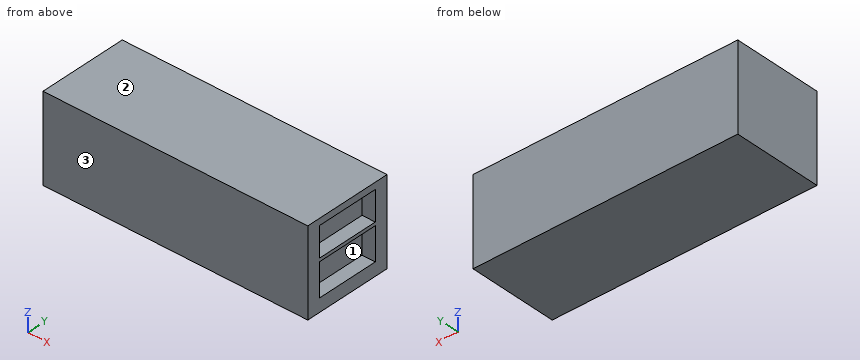
from build123d import *

# Parameters (mm, degrees)
F0_W     = 2032
F0_H     = 660.4
F1_DEPTH = 685.8
F2_W     = 482.6
F2_H     = 228.6
F2_H_2   = 254
F3_DEPTH = 101.6
F4_W     = 482.6
F4_H     = 254
F5_DEPTH = 101.6


with BuildPart() as f1:
    # F0 (on Front) → F1 (new body)
    with BuildSketch(Plane.XZ):
        with Locations((13.692988, -207.793446)):
            Rectangle(F0_W, F0_H)
    extrude(amount=F1_DEPTH)

    # F2 (on face) → F3 (cut)
    with BuildSketch(Plane.YZ.offset(1029.692988)):
        with Locations((-342.9, -42.693446)):
            Rectangle(F2_W, F2_H)
        with Locations((-342.9, -309.393446)):
            Rectangle(F2_W, F2_H_2)
    extrude(amount=-F3_DEPTH, mode=Mode.SUBTRACT)

    # F4 (on face) → F5 (join)
    with BuildSketch(Plane(origin=(-1002.307012, 0, 0), x_dir=(0, -1, 0), z_dir=(-1, 0, 0))):
        with Locations((342.9, -55.393446)):
            Rectangle(F4_W, F4_H)
        with Locations((342.9, -334.793446)):
            Rectangle(F4_W, F4_H)
    extrude(amount=-F5_DEPTH)


solid = f1.part
Geometry check sheet. Reference: the model listing, model coordinates, mm. Face numbers are marked on the shaded views. Round coordinates to 2 decimals unless told otherwise and drop trailing zeros. Order: outer loops, then holes, each group sorted by start corner. A loop starts at its lowest first (then second) coordinate and runs counter-clockwise, first axis right, second up. Notation, with made-up numbers: (52.25, 2.5) -> (64.25, 2.5) arc R32 cw to (64.25, 37.5) -> close; hole circle Ø6 at (27.25, 5.5). An arc over 180 degrees is marked (long way). Use one line per item in the form item = value.
1. Cross-section at B-B, the plane y = -561. Enter the section's corners in (x, z).
Working result:
outline = (-1002.31, -537.99) -> (1029.69, -537.99) -> (1029.69, -436.39) -> (928.09, -436.39) -> (928.09, -182.39) -> (1029.69, -182.39) -> (1029.69, -156.99) -> (928.09, -156.99) -> (928.09, 71.61) -> (1029.69, 71.61) -> (1029.69, 122.41) -> (-1002.31, 122.41) -> close
2. Mould release check, pull along Y, two halves, no side actions. Record for the marked faces 1, 2 and 3: pulls with the +Y half, pulls with the -Y half, needs draft (parallel to the pull), parting line crosses it, or undercut.
Working result:
face_1 = undercut
face_2 = needs draft
face_3 = pulls with the -Y half
3. Cross-section at A-A, the plane z = -240.5. Enter the section's corners in (x, y), plus the area to 3 significant figures.
Working result:
outline = (-1002.31, -685.8) -> (1029.69, -685.8) -> (1029.69, -584.2) -> (928.09, -584.2) -> (928.09, -101.6) -> (1029.69, -101.6) -> (1029.69, 0) -> (-1002.31, 0) -> close
area = 1,340,000 mm^2
4. Scan lines: line 1 along Z through (x, y) = (940.5, -138.5); line 2 along X through (y, z) = (-306, -322.5). Record each from-to range of solid material in increasing order. Write a range as from..to.
Working result:
line_1 = -537.99..-436.39, -182.39..-156.99, 71.61..122.41
line_2 = -1002.31..928.09
